```python
from build123d import *

# Parameters (mm, degrees)
SKETCH_1_W          = 25
SKETCH_1_H          = 8
EXTRUDE_1_DEPTH     = 8
SKETCH_2_R          = 1.5
CUT_EXTRUDE_1_DEPTH = 8
SKETCH_3_R          = 1.5
CUT_EXTRUDE_2_DEPTH = 8


with BuildPart() as part:
    # 草图1 → 凸台-拉伸1 (new body)
    with BuildSketch(Plane(origin=(0, 0, 0), x_dir=(1, 0, 0), z_dir=(0, 1, 0))):
        Rectangle(SKETCH_1_W, SKETCH_1_H)
    extrude(amount=EXTRUDE_1_DEPTH)

    # 草图2 → 切除-拉伸1 (cut)
    with BuildSketch(Plane(origin=(0, 8, 0), x_dir=(1, 0, 0), z_dir=(0, 1, 0))):
        with Locations(Location((7.5, 0, 0), (0, 0, 270))):
            Circle(SKETCH_2_R)
        with Locations(Location((-2.5, 0, 0), (0, 0, 270))):
            Circle(SKETCH_2_R)
    extrude(amount=-CUT_EXTRUDE_1_DEPTH, mode=Mode.SUBTRACT)

    # 草图3 → 切除-拉伸2 (cut)
    with BuildSketch(Plane.XY.offset(4)):
        with Locations((-7.5, 4)):
            Circle(SKETCH_3_R)
        with Locations((2.5, 4)):
            Circle(SKETCH_3_R)
    extrude(amount=-CUT_EXTRUDE_2_DEPTH, mode=Mode.SUBTRACT)


solid = part.part
```
Geometry check sheet. Reference: the model listing, model coordinates, mm. Coordinates: 2 decimals unless noted, no trailing zeros. Order: outer loops, then holes, each group sorted by start corner. A loop starts at its lowest first (then second) coordinate and runs counter-clockwise, first axis right, second up.
Item 1: Section check A-A (z = 0). Enter the section's corners in (x, y), plus the area to 3 significant figures.
Item 2: Scan lines: line 1 along X through (y, z) = (6.5, 0); line 2 along Y through (x, z) = (2.5, 1.5); line 3 along X through (y, z) = (4.75, 0.5). Record each from-to range of solid material in increasing order.
Item 3: Section check C-C (y = 2). Enter the section's corners in (x, z), plus the area to 3 significant figures.
Item 4: Mould release check, pull along Y, two halves, no side actions. Record for faces 1 (the cylindrical face through (1.39, 5.01, 0.06)), 2 (the cylindrical face through (6, 4, 0)), 3 (the flat face through (0, 8, 0)), 4 (the flat face through (0, 0, 0)): released by +Y, released by -Y, zero draft, split by the parting line, or undercut.
Item 5: Depth check by flat-ended pin: pin 1 (4 mm diameter, centred on x = 2, y = 5, fed in from +Z). Enter the tip coordinate at first touch or a pass-through.
Item 6: Section check D-D (z = 3). Enter the section's corners in (x, y).
Item 7: Section check B-B (x = -2.5). Enter the section's corners in (y, z), plus the area to 3 significant figures.
Check sheet entries:
1. outline: (-12.5, 0) - (-4, 0) - (-4, 8) - (-12.5, 8) - close; (-1, 0) - (6, 0) - (6, 8) - (-1, 8) - close; (9, 0) - (12.5, 0) - (12.5, 8) - (9, 8) - close; hole circle Ø3 at (-7.5, 4); hole circle Ø3 at (2.5, 4)
1. area: 138 mm2
2. line 1: x = -12.5 to -4, -1 to 6, 9 to 12.5
2. line 2: y = 0 to 2.5, 5.5 to 8
2. line 3: x = -12.5 to -8.8, -6.2 to -3.91, -1.09 to 1.2, 3.8 to 6.09, 8.91 to 12.5
3. outline: (-12.5, -4) - (12.5, -4) - (12.5, 4) - (-12.5, 4) - close; hole circle Ø3 at (-2.5, 0); hole circle Ø3 at (7.5, 0)
3. area: 186 mm2
4. face 1: undercut
4. face 2: zero draft
4. face 3: released by +Y
4. face 4: released by -Y
5. pin 1: stops at z = 4
6. outline: (-12.5, 0) - (12.5, 0) - (12.5, 8) - (-12.5, 8) - close; hole circle Ø3 at (-7.5, 4); hole circle Ø3 at (2.5, 4)
7. outline: (0, -4) - (8, -4) - (8, -1.5) - (0, -1.5) - close; (0, 1.5) - (8, 1.5) - (8, 4) - (0, 4) - close
7. area: 40.0 mm2
